from build123d import *

# Parameters (mm, degrees)
SKETCH_W        = 105.8
SKETCH_H        = 81.3
SKETCH_W_2      = 5
SKETCH_H_2      = 4
PAD_DEPTH       = 1
SKETCH001_W     = 105.8
SKETCH001_H     = 81.3
SKETCH001_W_2   = 83.934342
SKETCH001_H_2   = 64.581907
SKETCH001_W_3   = 2.8
SKETCH001_H_3   = 1.8
PAD001_DEPTH    = 1
SKETCH002_R     = 0.9
PAD002_DEPTH    = 4
SKETCH003_W     = 105.8
SKETCH003_H     = 81.3
SKETCH003_W_2   = 103.8
SKETCH003_H_2   = 79.3
PAD003_DEPTH    = 3
SKETCH014_W     = 5
SKETCH014_H     = 4
POCKET001_DEPTH = 0.5
SKETCH028_W     = 88.334342
SKETCH028_H     = 68.981907
SKETCH028_W_2   = 84.334342
SKETCH028_H_2   = 64.981907
POCKET015_DEPTH = 0.8


with BuildPart() as part:
    # Sketch (on Face286 of Binder) → Pad (new body)
    with BuildSketch(Plane.XY.offset(0.85)):
        Rectangle(SKETCH_W, SKETCH_H)
        Polygon((-45.8999, -39.65), (45.8999, -39.65), (45.8999, 38.9351), (-45.8999, 38.9351), (-45.8999, 10.824213), (-50.377559, 10.824213), (-50.377559, -10.886816), (-45.8999, -10.886816), align=None, mode=Mode.SUBTRACT)
        with Locations((48.4, 36.15)):
            Rectangle(SKETCH_W_2, SKETCH_H_2, mode=Mode.SUBTRACT)
    extrude(amount=PAD_DEPTH)

    # Sketch001 (on Face18 of Pad) → Pad001 (join)
    with BuildSketch(Plane.XY.offset(1.85)):
        Rectangle(SKETCH001_W, SKETCH001_H)
        with Locations((0, 3.16961)):
            Rectangle(SKETCH001_W_2, SKETCH001_H_2, mode=Mode.SUBTRACT)
        with Locations((48.4, 36.15)):
            Rectangle(SKETCH001_W_3, SKETCH001_H_3, mode=Mode.SUBTRACT)
    extrude(amount=PAD001_DEPTH)

    # Sketch002 (on Face1 of Pad001) → Pad002 (join)
    with BuildSketch(Plane(origin=(0, 0, 0.85), x_dir=(1, 0, 0), z_dir=(0, 0, -1))):
        with Locations((-48.4, 36.15)):
            Circle(SKETCH002_R)
        with Locations((48.4, 36.15)):
            Circle(SKETCH002_R)
        with Locations((-48.4, -36.15)):
            Circle(SKETCH002_R)
    extrude(amount=PAD002_DEPTH)

    # Sketch003 (on Face1 of Pad002) → Pad003 (join)
    with BuildSketch(Plane(origin=(0, 0, 0.85), x_dir=(1, 0, 0), z_dir=(0, 0, -1))):
        Rectangle(SKETCH003_W, SKETCH003_H)
        Rectangle(SKETCH003_W_2, SKETCH003_H_2, mode=Mode.SUBTRACT)
    extrude(amount=PAD003_DEPTH)

    # Sketch014 (on Face24 of Pad003) → Pocket001 (cut)
    with BuildSketch(Plane(origin=(0, 0, 1.85), x_dir=(1, 0, 0), z_dir=(0, 0, -1))):
        with Locations((48.4, -36.15)):
            Rectangle(SKETCH014_W, SKETCH014_H)
    extrude(amount=-POCKET001_DEPTH, mode=Mode.SUBTRACT)

    # Sketch028 (on Face19 of Pocket001) → Pocket015 (cut)
    with BuildSketch(Plane(origin=(0, 0, 1.85), x_dir=(1, 0, 0), z_dir=(0, 0, -1))):
        with Locations((0, -3.169609)):
            Rectangle(SKETCH028_W, SKETCH028_H)
        with Locations((0, -3.169609)):
            Rectangle(SKETCH028_W_2, SKETCH028_H_2, mode=Mode.SUBTRACT)
    extrude(amount=-POCKET015_DEPTH, mode=Mode.SUBTRACT)


solid = part.part
Input: part model. Units: mm. Frame: model coordinates. A direction names the side the tool comes from. Coordinates: 2 decimals unless noted, no trailing zeros. Loops run counter-clockwise (first coordinate to the right, second up) from the corner with the lowest first, then second, coordinate; pieces in that order, holes last.
Q1. Cut plane A-A (z = -0.1). Output: boundary loops of the cut face in (x, y).
Q2. Set-up query: faces 1 (the face through (-52.9, 1, 0)), 2 (the face through (-46.4, -11.6, 0.85)). Return all of +Z, -Z, +X, -X, +Y, -Y with unobstructed straight access to the full face (end or side cutting, diameter ignored); none if empty.
Q3. Cut plane B-B (y = 1). Output: boundary loops of the cut face in (x, z), then the cut area to 3 significant figures.
Q4. Material intervals for line 1 (Y direction, x = 27, z = 2.4); line 2 (X direction, y = -31, z = 0.15); line 3 (Y direction, x = 10, z = -2.05), sorted ascending.
Q5. Cut plane D-D (y = 23). Output: boundary loops of the cut face in (x, z), then the cut area to 3 significant figures.
Q6. Draft query along X for faces 3 (the face through (52.9, 1, 0)), 4 (the face through (-13, -32, 1.85)), 5 (the face through (-3, 36, 2.65)), 6 (the face through (-1, -40.65, 0)). Return one class per face: +X half, -X half, draft (parallel to the pull), parting line (faces both ways), or undercut.
Q7. Cut plane C-C (x = -17). Output: boundary loops of the cut face in (y, z), then the cut area to 3 significant figures.
Working result:
1. outline: (-52.9, -40.65) - (52.9, -40.65) - (52.9, 40.65) - (-52.9, 40.65) - close; circle Ø1.8 at (-48.4, -36.15); circle Ø1.8 at (-48.4, 36.15); circle Ø1.8 at (48.4, -36.15); hole (-51.9, -39.65) - (51.9, -39.65) - (51.9, 39.65) - (-51.9, 39.65) - close
2. face 1: +Z, -Z, -X, +Y, -Y
2. face 2: -Z
3. outline: (-52.9, -2.15) - (-51.9, -2.15) - (-51.9, 0.85) - (-50.38, 0.85) - (-50.38, 1.85) - (-44.17, 1.85) - (-44.17, 2.65) - (-42.17, 2.65) - (-42.17, 1.85) - (-41.97, 1.85) - (-41.97, 2.85) - (-52.9, 2.85) - close; (41.97, 1.85) - (42.17, 1.85) - (42.17, 2.65) - (44.17, 2.65) - (44.17, 1.85) - (45.9, 1.85) - (45.9, 0.85) - (51.9, 0.85) - (51.9, -2.15) - (52.9, -2.15) - (52.9, 2.85) - (41.97, 2.85) - close
3. area: 34.2 mm2
4. line 1: y = -40.65 to -31.32, -29.32 to -29.12, 35.46 to 35.66, 37.66 to 40.65
4. line 2: x = -52.9 to -51.9, 51.9 to 52.9
4. line 3: y = -40.65 to -39.65, 39.65 to 40.65
5. outline: (-52.9, -2.15) - (-51.9, -2.15) - (-51.9, 0.85) - (-45.9, 0.85) - (-45.9, 1.85) - (-44.17, 1.85) - (-44.17, 2.65) - (-42.17, 2.65) - (-42.17, 1.85) - (-41.97, 1.85) - (-41.97, 2.85) - (-52.9, 2.85) - close; (41.97, 1.85) - (42.17, 1.85) - (42.17, 2.65) - (44.17, 2.65) - (44.17, 1.85) - (45.9, 1.85) - (45.9, 0.85) - (51.9, 0.85) - (51.9, -2.15) - (52.9, -2.15) - (52.9, 2.85) - (41.97, 2.85) - close
5. area: 38.7 mm2
6. face 3: +X half
6. face 4: undercut
6. face 5: undercut
6. face 6: draft
7. outline: (-40.65, -2.15) - (-39.65, -2.15) - (-39.65, 1.85) - (-31.32, 1.85) - (-31.32, 2.65) - (-29.32, 2.65) - (-29.32, 1.85) - (-29.12, 1.85) - (-29.12, 2.85) - (-40.65, 2.85) - close; (35.46, 1.85) - (35.66, 1.85) - (35.66, 2.65) - (37.66, 2.65) - (37.66, 1.85) - (38.94, 1.85) - (38.94, 0.85) - (39.65, 0.85) - (39.65, -2.15) - (40.65, -2.15) - (40.65, 2.85) - (35.46, 2.85) - close
7. area: 22.2 mm2
